Part print with two shaded views. Sizes in mm from the minimum x, y, z corner. A direction names the side the tool comes from. Round coordinates to 2 decimals unless told otherwise and drop trailing zeros. Write each loop counter-clockwise with the first axis right and the second up, starting at its lowest first coordinate (ties: lowest second). Pieces come first, ordered by that corner, then holes. Notation, with made-up numbers: (-21, 59.5) -> (5, 59.5) arc R27 ccw to (5, 98.5) -> close; hole circle Ø8 at (30.5, 63.5). An arc over 180 degrees is marked (long way). Answer in a Markdown table with one row per item. Add a question column.
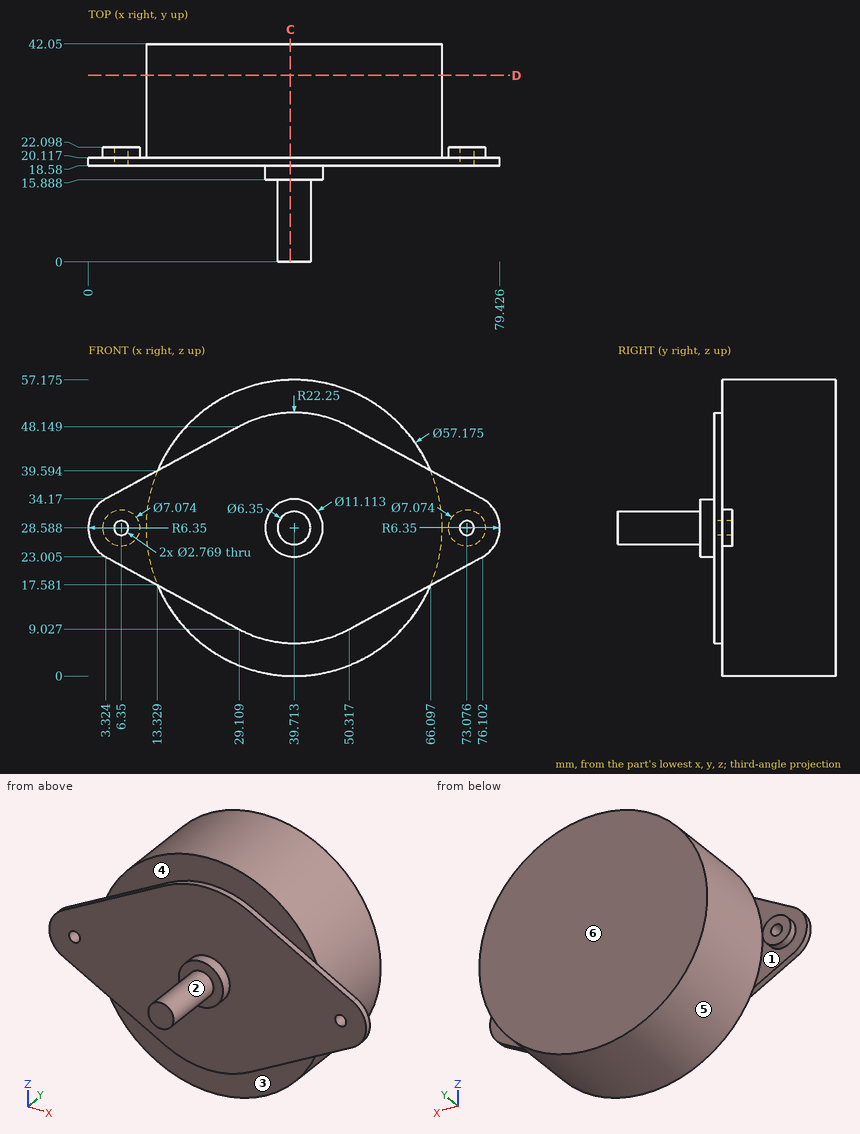
Item 1: Tool access for the marked faces 4, 5 and 6: list every direction of +Z, -Z, +X, -X, +Y, -Y with a clear straight run to the whole face (end or side of a thin tool).
Item 2: Drill centre lines: probe 1 along Y at (x, z) = (55, 49); probe 2 along Y at (x, z) = (40, 36.5); probe 3 along Z at (x, y) = (6, 21). Where is each one in solid material? Low to high.
Item 3: Pin check, flat tips, straight feed: pin 1 (4 mm diameter, centred on x = 75, z = 23.5, fed in from +Y); pin 2 (9 mm diameter, centred on x = 37, z = 13, fed in from -Y); pin 3 (3 mm diameter, centred on x = 32.5, y = 27, fed in from -Z). Stop position of each tip, or through.
Item 4: Saw through at C-C on x = 39. Give the cut face in (y, z).
Item 5: Saw through at D-D on y = 36. Give the cut face in (x, z) (1 decimal), then the cut area to 3 significant figures.
Item 6: Two-plate mould, pull along X, no slides. Class the marked faces 1, 2 and 3: +X half, -X half, draft (parallel to the pull), parting line (faces both ways), or undercut.
Recorded:
| question | item | result |
|---|---|---|
| 1 | face 4 | +Z, -Y |
| 1 | face 5 | +Y |
| 1 | face 6 | +Z, -Z, +X, -X, +Y |
| 2 | probe 1 | 20.12 to 42.05 |
| 2 | probe 2 | 18.58 to 42.05 |
| 2 | probe 3 | 25.07 to 27.25, 29.93 to 32.11 |
| 3 | pin 1 | y = 22.1 |
| 3 | pin 2 | y = 18.58 |
| 3 | pin 3 | z = 0.58 |
| 4 | outline | (0, 25.49) -> (15.89, 25.49) -> (15.89, 23.08) -> (18.58, 23.08) -> (18.58, 6.35) -> (20.12, 6.35) -> (20.12, 0.01) -> (42.05, 0.01) -> (42.05, 57.17) -> (20.12, 57.17) -> (20.12, 50.83) -> (18.58, 50.83) -> (18.58, 34.1) -> (15.89, 34.1) -> (15.89, 31.68) -> (0, 31.68) -> close |
| 5 | outline | circle Ø57.2 at (39.7, 28.6) |
| 5 | area | 2,570 mm2 |
| 6 | face 1 | undercut |
| 6 | face 2 | parting line |
| 6 | face 3 | draft |
